Check sheet for the drawn part. Datum: minimum x, y, z corner. Units: mm. A direction names the side the tool comes from. Coordinates: 2 decimals unless noted, no trailing zeros. Write each loop counter-clockwise with the first axis right and the second up, starting at its lowest first coordinate (ties: lowest second). Pieces come first, ordered by that corner, then holes. Notation, with made-up numbers: (2, 10) -> (48, 10) arc R32 cw to (48, 36) -> close; hole circle Ø8 at (-9, 70). An arc over 180 degrees is marked (long way). One line per question, with ' | ' between items.
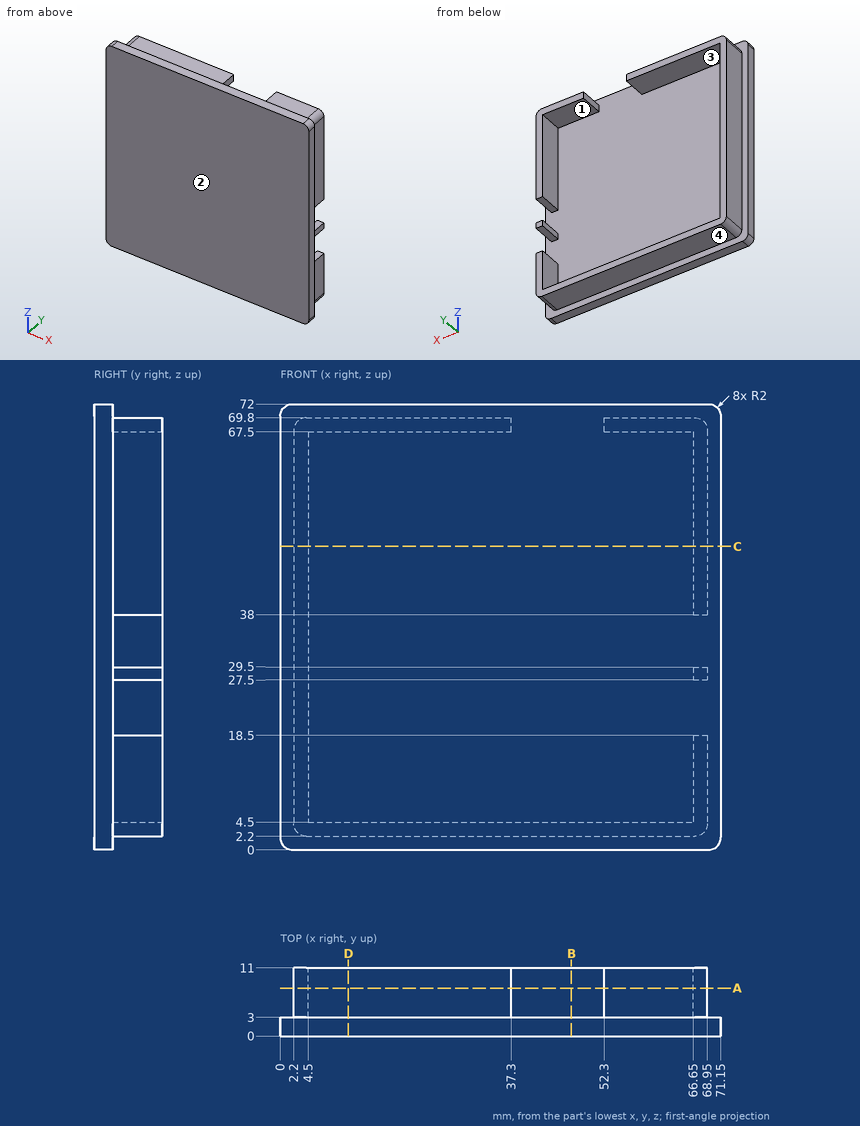
1. Cross-section at C-C on z = 49. Record the boundary of the cut face in (x, y), and give its area (3 significant figures).
Worked answers:
outline: (0, 0) -> (71.15, 0) -> (71.15, 3) -> (68.95, 3) -> (68.95, 11) -> (66.65, 11) -> (66.65, 3) -> (4.5, 3) -> (4.5, 11) -> (2.2, 11) -> (2.2, 3) -> (0, 3) -> close | area: 250 mm²
2. Cross-section at D-D on x = 11. Record the boundary of the cut face in (y, z), and give its area (3 significant figures).
Worked answers:
outline: (0, 0) -> (3, 0) -> (3, 2.2) -> (11, 2.2) -> (11, 4.5) -> (3, 4.5) -> (3, 67.5) -> (11, 67.5) -> (11, 69.8) -> (3, 69.8) -> (3, 72) -> (0, 72) -> close | area: 253 mm²
3. Go/stop test with flat-tipped pins: P1, Ø2.5, axis at x = 67.5, y = 9, coming from the +Z side; P2, Ø6, axis at x = 50.5, z = 19.5, coming from the +Y side; P3, Ø1.8, axis at x = 67.5, y = 7.5, coming from the -Z side. Record where each tip stops, or that it passes through.
Worked answers:
P1: z = 69.8 | P2: y = 3 | P3: z = 2.2
4. Material ranges on line 1 (X direction, y = 5.75, z = 28); line 2 (Z direction, x = 53, y = 8.25); line 3 (Y direction, x = 48, z = 58), recorded low to high. Write a range as from..to.
Worked answers:
line 1: 2.2..4.5, 66.65..68.95 | line 2: 2.2..4.5, 67.5..69.8 | line 3: 0..3
5. Tool access check on the marked faces 1 and 2. Record the directions out of +Z, -Z, +X, -X, +Y, -Y that give a thin tool (end or side, any length) a straight path to the whole face; none if there is none.
Worked answers:
face 1: +Y | face 2: +Z, -Z, +X, -X, -Y
6. Cross-section at B-B on x = 47. Record the boundary of the cut face in (y, z), and give its area (3 significant figures).
Worked answers:
outline: (0, 0) -> (3, 0) -> (3, 2.2) -> (11, 2.2) -> (11, 4.5) -> (3, 4.5) -> (3, 72) -> (0, 72) -> close | area: 234 mm²
7. Cross-section at A-A on y = 7.75. Record the boundary of the cut face in (x, z), and give its area (3 significant figures).
Worked answers:
outline: (2.2, 4.2) arc R2 ccw to (4.2, 2.2) -> (66.95, 2.2) arc R2 ccw to (68.95, 4.2) -> (68.95, 18.5) -> (66.65, 18.5) -> (66.65, 4.5) -> (4.5, 4.5) -> (4.5, 67.5) -> (37.3, 67.5) -> (37.3, 69.8) -> (4.2, 69.8) arc R2 ccw to (2.2, 67.8) -> close; (52.3, 67.5) -> (66.65, 67.5) -> (66.65, 38) -> (68.95, 38) -> (68.95, 67.8) arc R2 ccw to (66.95, 69.8) -> (52.3, 69.8) -> close; (66.65, 27.5) -> (68.95, 27.5) -> (68.95, 29.5) -> (66.65, 29.5) -> close | area: 519 mm²
8. Mould release check, pull along X, two halves, no side actions. Record for the marked faces 3 and 4: released by +X, released by -X, zero draft, split by the parting line, or undercut.
Worked answers:
face 3: undercut | face 4: zero draft
